Read the model definition and answer for the solid it produces. Units are mm, in the model's axes. A direction names the side the tool comes from. Coordinates: 2 decimals unless noted, no trailing zeros. Write each loop counter-clockwise with the first axis right and the second up, starting at its lowest first coordinate (ties: lowest second). Pieces come first, ordered by that corner, then holes.
(1) The part is cut by section C-C, the plane y = -8. Determine the outline of the cut face in (x, z), and give its area (3 significant figures).
(2) Determine the mould class of faces 4 (the flat face through (0, 38, 13)), 5 (the flat face through (13, 25.4, 38)), 6 (the flat face through (0, -13, 13)) for opening direction X: pulls with the +X half, pulls with the -X half, needs draft (parallel to the pull), parting line crosses it, or undercut.
(3) Which of the six approach directions +Z, -Z, +X, -X, +Y, -Y give full straight-line access (tool end or side, diameter ignored) to faces 1 (the flat face through (13, 38, 25.4)), 2 (the flat face through (0, 13, 38)), 3 (the flat face through (-13, 25.4, 13))?
(4) Straight lines are drawn through the part: line 1 along X through (y, z) = (-18, 13); line 2 along Y through (x, z) = (6, 2); line 3 along X through (y, z) = (6, 26.5). For each, find the intervals that lie inside material, in ascending order.
(5) The part is cut by section D-D, the plane x = 2. Determine the outline of the cut face in (y, z).
(6) Given pin 1 (7.5 mm diameter, centred on x = -15.5, z = 18, fed in from +Y); pin 2 (12.5 mm diameter, centred on x = -14, y = -8, fed in from +Z); pin 3 (12.5 mm diameter, centred on y = 39, z = 17.5, fed in from -X); pin 4 (10 mm diameter, centred on x = -2, y = 4.5, fed in from +Z), each flat-ended and moving along its own axis, determine where each tip first touches the part or whether it passes through.
(7) The part is cut by section A-A, the plane z = 10.5. Determine the outline of the cut face in (x, y).
(8) The part is cut by section B-B, the plane x = -14.5. Determine the outline of the cut face in (y, z), and give its area (3 significant figures).
```python
from build123d import *

# Parameters (mm, degrees)
F0_W     = 25.400002
F0_H     = 25.4
F0_W_2   = 25.4
F1_DEPTH = 25.4
F2_W     = 25.4
F2_H     = 25.4
F3_DEPTH = 25.4


with BuildPart() as f1:
    # F0 (on Top) → F1 (new body)
    with BuildSketch(Plane.XY):
        with Locations((-12.700001, -12.7)):
            Rectangle(F0_W, F0_H)
        with Locations((12.7, 12.7)):
            Rectangle(F0_W_2, F0_H)
        with Locations((-12.700001, 12.7)):
            Rectangle(F0_W, F0_H)
        with Locations((12.7, 38.1)):
            Rectangle(F0_W_2, F0_H)
    extrude(amount=F1_DEPTH)

    # F2 (on Right) → F3 (join)
    with BuildSketch(Plane.YZ):
        with Locations((12.7, 37.954024)):
            Rectangle(F2_W, F2_H)
    extrude(amount=F3_DEPTH)


solid = f1.part
```
Computed:
1. outline: (-25.4, 0) - (0, 0) - (0, 25.4) - (-25.4, 25.4) - close
1. area: 645 mm2
2. face 4: pulls with the -X half
2. face 5: needs draft
2. face 6: pulls with the +X half
3. face 1: +Z, +X, -X, +Y
3. face 2: +Z, -X, +Y, -Y
3. face 3: +Z, -Z, -X, +Y
4. line 1: x = -25.4 to 0
4. line 2: y = 0 to 50.8
4. line 3: x = 0 to 25.4
5. outline: (0, 0) - (50.8, 0) - (50.8, 25.4) - (25.4, 25.4) - (25.4, 50.65) - (0, 50.65) - close
6. pin 1: stops at y = 25.4
6. pin 2: stops at z = 25.4
6. pin 3: stops at x = 0
6. pin 4: stops at z = 50.65
7. outline: (-25.4, -25.4) - (0, -25.4) - (0, 0) - (25.4, 0) - (25.4, 50.8) - (0, 50.8) - (0, 25.4) - (-25.4, 25.4) - close
8. outline: (-25.4, 0) - (25.4, 0) - (25.4, 25.4) - (-25.4, 25.4) - close
8. area: 1,290 mm2
